Here's how the part is built. I have some questions about the finished solid (model axes, mm). A direction names the side the tool comes from. Coordinates: 2 decimals unless noted, no trailing zeros. Write each loop counter-clockwise with the first axis right and the second up, starting at its lowest first coordinate (ties: lowest second). Pieces come first, ordered by that corner, then holes.
Item 1: For faces 1 (the face through (14.7, 0.3, 37)), 2 (the face through (46, 0, 41)), 3 (the face through (107, 19, 22.5)), 4 (the face through (107.5, 29, 0)), 5 (the face through (108, 19, -22.5)), which set-ups out of +Z, -Z, +X, -X, +Y, -Y let a thin tool reach every point of the face, with its end or its side?
Item 2: I want a section at B-B (y = -18). Please give me the cut outline in (x, z), and give its area (3 significant figures).
Item 3: I want a section at A-A (x = 48). Please give me the cut outline in (y, z), and give its area (3 significant figures).
Item 4: I'm going to push flat-ended pins straight in: P1, Ø7.5, axis at x = 107, y = 15, coming from the -Z side; P2, Ø8, axis at x = 49.5, z = 35.5, coming from the -Y side; P3, Ø12, axis at x = 30, y = 0, coming from the +Z side. Where does each tip first touch, or does it pass through?
Item 5: I want a section at D-D (x = 23). Please give me the cut outline in (y, z).
Item 6: If we mould it in two halves opening along Z, with no side actions, what happens to faces 6 (the face through (107, 41, -42)), 7 (the face through (107.72, 41.056, 27.505)), 8 (the face through (110.1, 37, 27.8))? For each: pulls with the +Z half, pulls with the -Z half, needs draft (parallel to the pull), parting line crosses it, or undercut.
Item 7: I want a section at C-C (z = -12.5). Please give me the cut outline in (x, y), and give its area (3 significant figures).
Item 8: Please list where these lines run through material, in increasing order: line 1 (X direction, y = 42.5, z = 32.5); line 2 (Y direction, x = 73, z = 0); line 3 (Y direction, x = 96.5, z = -2).
from build123d import *

# Parameters (mm, degrees)
SKETCH_1_R           = 22.5
SKETCH_1_R_2         = 15
EXTRUDE_1_DEPTH      = 120
EXTRUDE_START        = 45
SKETCH_2_W           = 25
SKETCH_2_H           = 19.5
SKETCH_2_R           = 5
SKETCH_2_W_2         = 12.5
SKETCH_2_H_2         = 15
EXTRUDE_5_DEPTH      = 8
EXTRUDE_6_REACH      = 173.867
EXTRUDE_6_END_RADIUS = 22.5
EXTRUDE_START_2      = 37
EXTRUDE_7_DEPTH      = 8
EXTRUDE_8_REACH      = 174.831
EXTRUDE_8_END_RADIUS = 22.5
CUT_EXTRUDE_1_REACH  = 137.831
SKETCH_3_4_R         = 10
CUT_EXTRUDE_2_REACH  = 156.9
SKETCH_4_R           = 2


with BuildPart() as part:
    # Sketch 1 → Extrude 1 (new body)
    with BuildSketch(Plane(origin=(0, 0, 0), x_dir=(0, 0, -1), z_dir=(1, 0, 0))):
        Circle(SKETCH_1_R)
        Circle(SKETCH_1_R_2, mode=Mode.SUBTRACT)
    extrude(amount=EXTRUDE_1_DEPTH)



with BuildPart() as body_2:
    # Sketch 2 → Extrude 5 (new body)
    # profile 1 of 6: a face of its own
    with BuildSketch(Plane(origin=(0, 0, 0), x_dir=(1, 0, 0), z_dir=(0, 1, 0)).offset(EXTRUDE_START)):
        Polygon((107.5, 0), (120, 0), (120, 22.5), (95, 22.5), (95, 15), (107.5, 15), align=None)
    # profile 2 of 6: a face of its own
    with BuildSketch(Plane(origin=(0, 0, 0), x_dir=(1, 0, 0), z_dir=(0, 1, 0)).offset(EXTRUDE_START)):
        Polygon((95, -22.5), (120, -22.5), (120, 0), (107.5, 0), (107.5, -15), (95, -15), align=None)
    # profile 3 of 6: a face of its own
    with BuildSketch(Plane(origin=(0, 0, 0), x_dir=(1, 0, 0), z_dir=(0, 1, 0)).offset(EXTRUDE_START)):
        with Locations((107.5, -32.25)):
            Rectangle(SKETCH_2_W, SKETCH_2_H)
        with Locations(Location((107.5, -32.5, 0), (0, 0, 270))):
            Circle(SKETCH_2_R, mode=Mode.SUBTRACT)
    # profile 4 of 6: a face of its own
    with BuildSketch(Plane(origin=(0, 0, 0), x_dir=(1, 0, 0), z_dir=(0, 1, 0)).offset(EXTRUDE_START)):
        with Locations((107.5, 32.25)):
            Rectangle(SKETCH_2_W, SKETCH_2_H)
        with Locations(Location((107.5, 32.5, 0), (0, 0, 270))):
            Circle(SKETCH_2_R, mode=Mode.SUBTRACT)
    # profile 5 of 6: a face of its own
    with BuildSketch(Plane(origin=(0, 0, 0), x_dir=(1, 0, 0), z_dir=(0, 1, 0)).offset(EXTRUDE_START)):
        with Locations((101.25, 7.5)):
            Rectangle(SKETCH_2_W_2, SKETCH_2_H_2)
    # profile 6 of 6: a face of its own
    with BuildSketch(Plane(origin=(0, 0, 0), x_dir=(1, 0, 0), z_dir=(0, 1, 0)).offset(EXTRUDE_START)):
        with Locations((101.25, -7.5)):
            Rectangle(SKETCH_2_W_2, SKETCH_2_H_2)
    extrude(amount=-EXTRUDE_5_DEPTH)


with BuildPart() as part_1:
    add(part.part)

    add(body_2.part)  # Extrude 6 merges body 2
    # Extrude 6: up to this cylinder (the profile starts outside it)
    extrude_6_end = Plane(origin=(110.625, 0, 0), z_dir=(-1, 0, 0)) * Cylinder(EXTRUDE_6_END_RADIUS, 393.734, mode=Mode.PRIVATE)
    # Sketch 2_7 → Extrude 6 (add, up to the surface)
    with BuildSketch(Plane(origin=(0, 0, 0), x_dir=(1, 0, 0), z_dir=(0, 1, 0)).offset(EXTRUDE_START_2), mode=Mode.PRIVATE) as extrude_6_sk1:
        Polygon((95, -22.5), (120, -22.5), (120, 0), (107.5, 0), (107.5, -15), (95, -15), align=None)
    extrude_6_tool1 = extrude(extrude_6_sk1.sketch, amount=-EXTRUDE_6_REACH, mode=Mode.PRIVATE) - extrude_6_end
    add(extrude_6_tool1.solids().sort_by_distance((110.625, 37, 13.125))[0])
    # Sketch 2_7 → Extrude 6 (add, up to the surface)
    with BuildSketch(Plane(origin=(0, 0, 0), x_dir=(1, 0, 0), z_dir=(0, 1, 0)).offset(EXTRUDE_START_2), mode=Mode.PRIVATE) as extrude_6_sk2:
        Polygon((107.5, 0), (120, 0), (120, 22.5), (95, 22.5), (95, 15), (107.5, 15), align=None)
    extrude_6_tool2 = extrude(extrude_6_sk2.sketch, amount=-EXTRUDE_6_REACH, mode=Mode.PRIVATE) - extrude_6_end
    add(extrude_6_tool2.solids().sort_by_distance((110.625, 37, -13.125))[0])



with BuildPart() as body_2_2:
    # Sketch 3 → Extrude 7 (new body)
    with BuildSketch(Plane.XY.offset(EXTRUDE_START)):
        with BuildLine():
            ThreePointArc((15, 0), (30, 15), (45, 0))
            Line((45, 0), (52.5, 0))
            ThreePointArc((52.5, 0), (30, 22.5), (7.5, 0))
            Line((7.5, 0), (15, 0))
        make_face()
        with BuildLine():
            Line((52.5, 0), (45, 0))
            ThreePointArc((45, 0), (30, -15), (15, 0))
            Line((15, 0), (7.5, 0))
            ThreePointArc((7.5, 0), (30, -22.5), (52.5, 0))
        make_face()
        with BuildLine():
            ThreePointArc((15, 0), (30, 15), (45, 0))
            Line((45, 0), (52.5, 0))
            ThreePointArc((52.5, 0), (30, 22.5), (7.5, 0))
            Line((7.5, 0), (15, 0))
        make_face()
        with BuildLine():
            Line((52.5, 0), (45, 0))
            ThreePointArc((45, 0), (30, -15), (15, 0))
            Line((15, 0), (7.5, 0))
            ThreePointArc((7.5, 0), (30, -22.5), (52.5, 0))
        make_face()
        with BuildLine():
            ThreePointArc((20, 0), (30, 10), (40, 0))
            Line((40, 0), (45, 0))
            ThreePointArc((45, 0), (30, 15), (15, 0))
            Line((15, 0), (20, 0))
        make_face()
        with BuildLine():
            Line((45, 0), (40, 0))
            ThreePointArc((40, 0), (30, -10), (20, 0))
            Line((20, 0), (15, 0))
            ThreePointArc((15, 0), (30, -15), (45, 0))
        make_face()
        with BuildLine():
            ThreePointArc((20, 0), (30, 10), (40, 0))
            Line((40, 0), (45, 0))
            ThreePointArc((45, 0), (30, 15), (15, 0))
            Line((15, 0), (20, 0))
        make_face()
        with BuildLine():
            Line((45, 0), (40, 0))
            ThreePointArc((40, 0), (30, -10), (20, 0))
            Line((20, 0), (15, 0))
            ThreePointArc((15, 0), (30, -15), (45, 0))
        make_face()
    extrude(amount=-EXTRUDE_7_DEPTH)


with BuildPart() as part_2:
    add(part_1.part)

    add(body_2_2.part)  # Extrude 8 merges body 2 2
    # Extrude 8: up to this cylinder (the profile starts outside it)
    extrude_8_end = Plane(origin=(30, 0, 0), z_dir=(-1, 0, 0)) * Cylinder(EXTRUDE_8_END_RADIUS, 420.662, mode=Mode.PRIVATE)
    # Sketch 3_3 → Extrude 8 (add, up to the surface)
    with BuildSketch(Plane.XY.offset(EXTRUDE_START_2), mode=Mode.PRIVATE) as extrude_8_sk1:
        with BuildLine():
            ThreePointArc((20, 0), (30, 10), (40, 0))
            Line((40, 0), (45, 0))
            ThreePointArc((45, 0), (30, 15), (15, 0))
            Line((15, 0), (20, 0))
        make_face()
    extrude_8_tool1 = extrude(extrude_8_sk1.sketch, amount=-EXTRUDE_8_REACH, mode=Mode.PRIVATE) - extrude_8_end
    add(extrude_8_tool1.solids().sort_by_distance((17.5, 0.33541, 37))[0])
    # Sketch 3_3 → Extrude 8 (add, up to the surface)
    with BuildSketch(Plane.XY.offset(EXTRUDE_START_2), mode=Mode.PRIVATE) as extrude_8_sk2:
        with BuildLine():
            Line((45, 0), (40, 0))
            ThreePointArc((40, 0), (30, -10), (20, 0))
            Line((20, 0), (15, 0))
            ThreePointArc((15, 0), (30, -15), (45, 0))
        make_face()
    extrude_8_tool2 = extrude(extrude_8_sk2.sketch, amount=-EXTRUDE_8_REACH, mode=Mode.PRIVATE) - extrude_8_end
    add(extrude_8_tool2.solids().sort_by_distance((42.5, -0.33541, 37))[0])
    # Sketch 3_3 → Extrude 8 (add, up to the surface)
    with BuildSketch(Plane.XY.offset(EXTRUDE_START_2), mode=Mode.PRIVATE) as extrude_8_sk3:
        with BuildLine():
            ThreePointArc((20, 0), (30, 10), (40, 0))
            Line((40, 0), (45, 0))
            ThreePointArc((45, 0), (30, 15), (15, 0))
            Line((15, 0), (20, 0))
        make_face()
    extrude_8_tool3 = extrude(extrude_8_sk3.sketch, amount=-EXTRUDE_8_REACH, mode=Mode.PRIVATE) - extrude_8_end
    add(extrude_8_tool3.solids().sort_by_distance((17.5, 0.33541, 37))[0])
    # Sketch 3_3 → Extrude 8 (add, up to the surface)
    with BuildSketch(Plane.XY.offset(EXTRUDE_START_2), mode=Mode.PRIVATE) as extrude_8_sk4:
        with BuildLine():
            Line((45, 0), (40, 0))
            ThreePointArc((40, 0), (30, -10), (20, 0))
            Line((20, 0), (15, 0))
            ThreePointArc((15, 0), (30, -15), (45, 0))
        make_face()
    extrude_8_tool4 = extrude(extrude_8_sk4.sketch, amount=-EXTRUDE_8_REACH, mode=Mode.PRIVATE) - extrude_8_end
    add(extrude_8_tool4.solids().sort_by_distance((42.5, -0.33541, 37))[0])

    # Sketch 3_4 → Cut-Extrude 1 (cut, up to next)
    with BuildSketch(Plane.XY, mode=Mode.PRIVATE) as cut_extrude_1_sk1:
        with Locations((30, 0)):
            Circle(SKETCH_3_4_R)
    cut_extrude_1_tool1 = extrude(cut_extrude_1_sk1.sketch, amount=CUT_EXTRUDE_1_REACH, mode=Mode.PRIVATE) & part_2.part
    add(cut_extrude_1_tool1.solids().sort_by_distance((30, 0, 0))[0], mode=Mode.SUBTRACT)

    # Sketch 4 → Cut-Extrude 2 (cut, up to next)
    with BuildSketch(Plane.XY.offset(45), mode=Mode.PRIVATE) as cut_extrude_2_sk1:
        with Locations((30, 18)):
            Circle(SKETCH_4_R)
    cut_extrude_2_tool1 = extrude(cut_extrude_2_sk1.sketch, amount=-CUT_EXTRUDE_2_REACH, mode=Mode.PRIVATE) & part_2.part
    # Sketch 4 → Cut-Extrude 2 (cut, up to next)
    with BuildSketch(Plane.XY.offset(45), mode=Mode.PRIVATE) as cut_extrude_2_sk2:
        with Locations((48, 0)):
            Circle(SKETCH_4_R)
    cut_extrude_2_tool2 = extrude(cut_extrude_2_sk2.sketch, amount=-CUT_EXTRUDE_2_REACH, mode=Mode.PRIVATE) & part_2.part
    # Sketch 4 → Cut-Extrude 2 (cut, up to next)
    with BuildSketch(Plane.XY.offset(45), mode=Mode.PRIVATE) as cut_extrude_2_sk3:
        with Locations((30, -18)):
            Circle(SKETCH_4_R)
    cut_extrude_2_tool3 = extrude(cut_extrude_2_sk3.sketch, amount=-CUT_EXTRUDE_2_REACH, mode=Mode.PRIVATE) & part_2.part
    # Sketch 4 → Cut-Extrude 2 (cut, up to next)
    with BuildSketch(Plane.XY.offset(45), mode=Mode.PRIVATE) as cut_extrude_2_sk4:
        with Locations((12, 0)):
            Circle(SKETCH_4_R)
    cut_extrude_2_tool4 = extrude(cut_extrude_2_sk4.sketch, amount=-CUT_EXTRUDE_2_REACH, mode=Mode.PRIVATE) & part_2.part
    add(cut_extrude_2_tool1.solids().sort_by_distance((30, 18, 45))[0], mode=Mode.SUBTRACT)
    add(cut_extrude_2_tool2.solids().sort_by_distance((48, 0, 45))[0], mode=Mode.SUBTRACT)
    add(cut_extrude_2_tool3.solids().sort_by_distance((30, -18, 45))[0], mode=Mode.SUBTRACT)
    add(cut_extrude_2_tool4.solids().sort_by_distance((12, 0, 45))[0], mode=Mode.SUBTRACT)


solid = part_2.part
Answer:
1. face 1: none
1. face 2: +Z
1. face 3: +Z, +X, -Y
1. face 4: -X
1. face 5: -Z, +X, -X, -Y
2. outline: (0, -13.5) - (120, -13.5) - (120, 13.5) - (0, 13.5) - close; (16.5, 37) - (28, 37) - (28, 45) - (16.5, 45) - close; (32, 37) - (43.5, 37) - (43.5, 45) - (32, 45) - close
2. area: 3,420 mm2
3. outline: circle Ø45 at (0, 0); (-13.5, 37) - (-2, 37) - (-2, 45) - (-13.5, 45) - close; (2, 37) - (13.5, 37) - (13.5, 45) - (2, 45) - close; hole circle Ø30 at (0, 0)
3. area: 1,070 mm2
4. P1: stops at z = -22.5
4. P2: stops at y = -16.03
4. P3: stops at z = -13.75
5. outline: (-21.38, 37) - (-13.27, 37) - (-13.27, 18.17) arc R22.5 ccw (long way) to (13.27, 18.17) - (13.27, 37) - (21.38, 37) - (21.38, 45) - (7.14, 45) - (7.14, 13.19) arc R15 cw (long way) to (-7.14, 13.19) - (-7.14, 45) - (-21.38, 45) - close
6. face 6: pulls with the -Z half
6. face 7: undercut
6. face 8: needs draft
7. outline: (0, -18.71) - (120, -18.71) - (120, -8.29) - (0, -8.29) - close; (0, 8.29) - (120, 8.29) - (120, 45) - (95, 45) - (95, 37) - (107.5, 37) - (107.5, 18.71) - (0, 18.71) - close
7. area: 2,930 mm2
8. line 1: x = 95 to 102.5, 112.5 to 120
8. line 2: y = -22.5 to -15, 15 to 22.5
8. line 3: y = -22.41 to -14.87, 14.87 to 22.41, 37 to 45
